Geometry: see drawing. Coordinates: mm, zero at the bounding-box minimum. A direction names the side the tool comes from. Coordinates: 2 decimals unless noted, no trailing zeros. Loops run counter-clockwise (first coordinate to the right, second up) from the corner with the lowest first, then second, coordinate; pieces in that order, holes last. Notation, with made-up numbers: (-31.5, -35.5) -> (27.5, -35.5) arc R21 cw to (27.5, -5.5) -> close; hole circle Ø7 at (4.25, -28). An arc over 180 degrees is marked (long way). Answer as a JSON object with one key per item and string values.
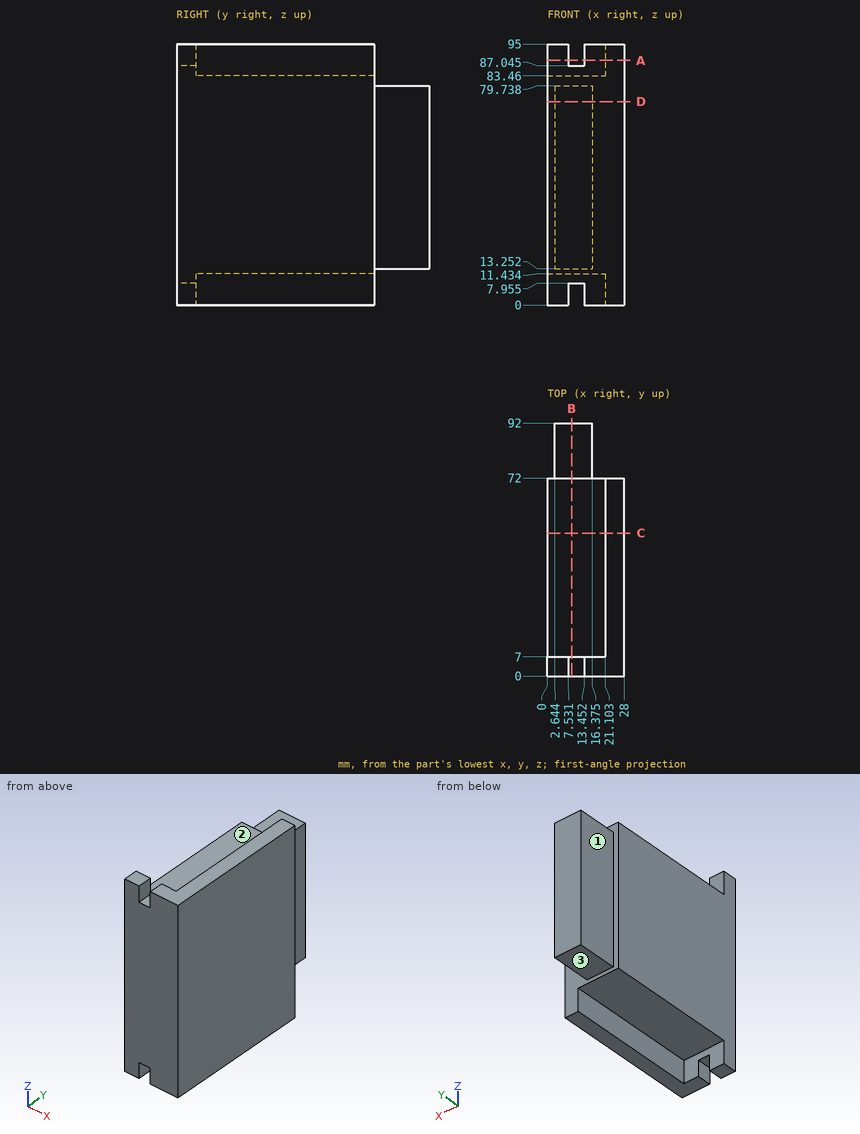
1. Section query C-C (y = 52). Return loops of the section in (x, z) (1 decimal).
Reply:
{"outline": "(0, 11.4) -> (21.1, 11.4) -> (21.1, 0) -> (28, 0) -> (28, 95) -> (21.1, 95) -> (21.1, 83.5) -> (0, 83.5) -> close"}
2. Section query D-D (z = 74). Return loops of the section in (x, y) (1 decimal), plus the area to 3 significant figures.
Reply:
{"outline": "(0, 0) -> (28, 0) -> (28, 72) -> (16.4, 72) -> (16.4, 92) -> (2.6, 92) -> (2.6, 72) -> (0, 72) -> close", "area": "2,290 mm2"}
3. Line query: line 1 along X through (y, z) = (81, 34.5) (1 decimal); line 2 along Z through (x, y) = (14.5, 81.5); line 3 along Y through (x, z) = (4, 80.5). Output: solid intervals per line, ascending.
Reply:
{"line 1": "x = 2.6 to 16.4", "line 2": "z = 13.25 to 79.74", "line 3": "y = 0 to 72"}
4. Section query B-B (x = 8.75). Return loops of the section in (y, z) (1 decimal), plus the area to 4 significant figures.
Reply:
{"outline": "(0, 8) -> (7, 8) -> (7, 11.4) -> (72, 11.4) -> (72, 13.3) -> (92, 13.3) -> (92, 79.7) -> (72, 79.7) -> (72, 83.5) -> (7, 83.5) -> (7, 87) -> (0, 87) -> close", "area": "6,565 mm2"}
5. Section query A-A (z = 89). Return loops of the section in (x, y), plus the area to 3 significant figures.
Reply:
{"outline": "(0, 0) -> (7.53, 0) -> (7.53, 7) -> (0, 7) -> close; (13.45, 0) -> (28, 0) -> (28, 72) -> (21.1, 72) -> (21.1, 7) -> (13.45, 7) -> close", "area": "603 mm2"}
6. Access query for the marked faces 1, 2 and 3. Directions: +Z, -Z, +X, -X, +Y, -Y. A direction counts if a zero-diameter tool reaches every point of the face in a straight line with its end or side. Return the directions, or none.
Reply:
{"face 1": "+Z, -Z, -X, +Y", "face 2": "+Z, -X, +Y", "face 3": "-Z, +X, -X, +Y"}
7. Pin query (flat end, axial travel): P1, Ø16, axis at y = 84, z = 53, coming from the -X side; P2, Ø6, axis at x = 15.5, y = 35, coming from the -Z side; P3, Ø1.5, axis at x = 19.5, z = 21, coming from the +Y side. Return the tip coordinate at first contact, or that it passes through.
Reply:
{"P1": "stops at x = 2.64", "P2": "stops at z = 11.43", "P3": "stops at y = 72"}
